from build123d import *

# Parameters (mm, degrees)
F0_W     = 30
F0_H     = 155
F1_DEPTH = 10
F2_R     = 5
F3_DEPTH = 10.001
F4_R     = 5


# Not quite as in the source:
# - a feature names something its author has since deleted; it is built from what else it names


with BuildPart() as f1:
    # F0 (on Front) → F1 (new body)
    with BuildSketch(Plane.XZ):
        Rectangle(F0_W, F0_H)
    extrude(amount=F1_DEPTH)

    # F2 (on face) → F3 (cut, through all)
    with BuildSketch(Plane.XZ.offset(10)):
        with Locations((0, 67.5)):
            Circle(F2_R)
    extrude(amount=-F3_DEPTH, mode=Mode.SUBTRACT)

    # F4
    f4_edges = [f1.edges().sort_by_distance(p)[0] for p in [
        (15, -5, 77.5),
        (-15, -5, 77.5),
    ]]
    fillet(f4_edges, radius=F4_R)


solid = f1.part
The listing builds one solid part. Answer for the finished solid, in the listing's coordinates (mm). Coordinates: 2 decimals unless noted, no trailing zeros. Order: outer loops, then holes, each group sorted by start corner. A loop starts at its lowest first (then second) coordinate and runs counter-clockwise, first axis right, second up.
Q1. A cutting plane is placed at B-B, the plane z = 67.5. Write down the section's boundary in (x, y).
Q2. A cutting plane is placed at C-C, the plane x = 0. Write down the section's boundary in (y, z), and give its area (3 significant figures).
Q3. For a pull along X with two mould halves and no side action, classify faces 1 (the face through (-13.57, -5.07, 76)), 2 (the face through (15, -5, -4)), 3 (the face through (2.688, -5.07, 71.716)), 4 (the face through (0, -5, -77.5)) as pulls with the +X half, pulls with the -X half, needs draft (parallel to the pull), parting line crosses it, or undercut.
Q4. Consider line 1 (Z direction, x = 0, y = -3.5); line 2 (Z direction, x = -1.5, y = -8.25); line 3 (Z direction, x = -11.5, y = -2). Determine where each line is inside the solid, lowest interval first.
Q5. A cutting plane is placed at A-A, the plane y = -5.5. Write down the section's boundary in (x, z).
Q6. Given P1, Ø9, axis at x = 0, z = 67.5, coming from the -Y side, flat-ended and moving along its own axis, determine where the tip first touches the part or whether it passes through.
Answers follow:
1. outline: (-15, -10) - (-5, -10) - (-5, 0) - (-15, 0) - close; (5, -10) - (15, -10) - (15, 0) - (5, 0) - close
2. outline: (-10, -77.5) - (0, -77.5) - (0, 62.5) - (-10, 62.5) - close; (-10, 72.5) - (0, 72.5) - (0, 77.5) - (-10, 77.5) - close
2. area: 1,450 mm2
3. face 1: pulls with the -X half
3. face 2: pulls with the +X half
3. face 3: undercut
3. face 4: needs draft
4. line 1: z = -77.5 to 62.5, 72.5 to 77.5
4. line 2: z = -77.5 to 62.73, 72.27 to 77.5
4. line 3: z = -77.5 to 77.27
5. outline: (-15, -77.5) - (15, -77.5) - (15, 72.5) arc R5 ccw to (10, 77.5) - (-10, 77.5) arc R5 ccw to (-15, 72.5) - close; hole circle Ø10 at (0, 67.5)
6. P1: passes through
